```python
from build123d import *

# Parameters (mm, degrees)
SKETCH1_R           = 4
BOSS_EXTRUDE1_DEPTH = 9


with BuildPart() as part:
    # Sketch1 → Boss-Extrude1 (new body)
    with BuildSketch(Plane(origin=(0, 0, 0), x_dir=(1, 0, 0), z_dir=(0, 1, 0))):
        Polygon((0, 62.5), (0, -62.5), (-30, -62.5), (-20, -27.5), (-20, 27.5), (-30, 62.5), align=None)
        with Locations(Location((-12.5, 47.5, 0), (0, 0, 270))):
            Circle(SKETCH1_R, mode=Mode.SUBTRACT)
        with Locations(Location((-12.5, -47.5, 0), (0, 0, 270))):
            Circle(SKETCH1_R, mode=Mode.SUBTRACT)
    extrude(amount=BOSS_EXTRUDE1_DEPTH)


solid = part.part
```
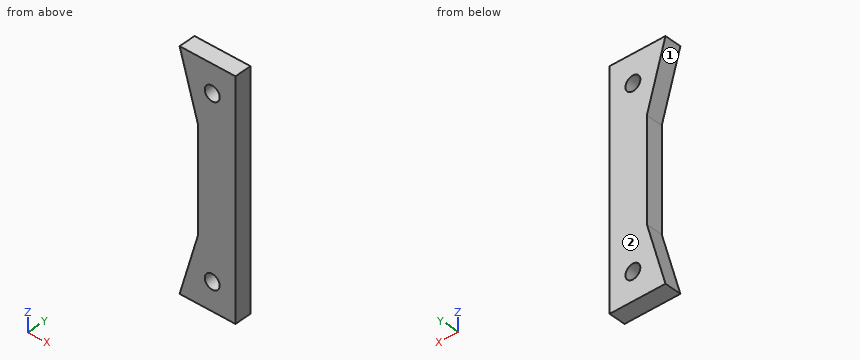
Geometry: final body of the model. Coordinates: model frame, mm. Face numbers are marked on the shaded views. Round coordinates to 2 decimals unless told otherwise and drop trailing zeros. Order: outer loops, then holes, each group sorted by start corner. A loop starts at its lowest first (then second) coordinate and runs counter-clockwise, first axis right, second up. Notation, with made-up numbers: (-7.5, 5.25) - (8.5, 5.25) arc R15 cw to (8.5, 12.25) - close; hole circle Ø1 at (-9, 68.25). An arc over 180 degrees is marked (long way). Use CSV: the item, a comma, the result in double quotes. Start each with the question number.
Q1. Mould query, pull axis Z, two halves, no side actions, for the marked faces 1 and 2. Classes: +Z half, -Z half, draft (parallel to the pull), parting line (faces both ways), or undercut.
Q2. First-contact query: pin 1 (4.5 mm diameter, centred on y = 3, z = 2, fed in from -X). Flat tip, straight axial feed; report the tip coordinate or a pass-through.
Q3. Section query D-D (z = -22). Return loops of the section in (x, y).
Q4. Section query C-C (z = 47.5). Return loops of the section in (x, y), and give its area (3 significant figures).
Q5. Section query A-A (x = -12.5). Return loops of the section in (y, z).
Q6. Material intervals for line 1 along X through (y, z) = (6.75, 47.5); line 2 along X through (y, z) = (5.75, -8); line 3 along X through (y, z) = (6.75, 42.5), sorted ascending. Write a range as from..to.
Q7. Section query B-B (y = 7.25). Return loops of the section in (x, z).
Result set:
1,face 1,"undercut"
1,face 2,"draft"
2,pin 1,"stops at x = -20"
3,outline,"(-20, 0) - (0, 0) - (0, 9) - (-20, 9) - close"
4,outline,"(-25.71, 0) - (-16.5, 0) - (-16.5, 9) - (-25.71, 9) - close; (-8.5, 0) - (0, 0) - (0, 9) - (-8.5, 9) - close"
4,area,"159 mm2"
5,outline,"(0, -62.5) - (9, -62.5) - (9, -51.5) - (0, -51.5) - close; (0, -43.5) - (9, -43.5) - (9, 43.5) - (0, 43.5) - close; (0, 51.5) - (9, 51.5) - (9, 62.5) - (0, 62.5) - close"
6,line 1,"x = -25.71..-16.5, -8.5..0"
6,line 2,"x = -20..0"
6,line 3,"x = -24.29..0"
7,outline,"(-30, -62.5) - (0, -62.5) - (0, 62.5) - (-30, 62.5) - (-20, 27.5) - (-20, -27.5) - close; hole circle Ø8 at (-12.5, -47.5); hole circle Ø8 at (-12.5, 47.5)"
